Autodesk Inventor part; units mm, degrees
ref_plane "YZ Plane" through (0, 0, 0) normal (1, 0, 0) x (0, 1, 0)
ref_plane "XZ Plane" through (0, 0, 0) normal (0, 1, 0) x (-1, 0, 0)
ref_plane "XY Plane" through (0, 0, 0) normal (0, 0, 1) x (1, 0, 0)
sketch "Sketch1" plane through (0, 0, 0) normal (1, 0, 0) x (0, 1, 0)
  line L0 (6.35, -3.6662) -> (0, -7.3323)
  line L1 (0, -7.3323) -> (-6.35, -3.6662)
  line L2 (-6.35, -3.6662) -> (-6.35, 3.6662)
  line L3 (-6.35, 3.6662) -> (0, 7.3323)
  line L4 (0, 7.3323) -> (6.35, 3.6662)
  line L5 (6.35, 3.6662) -> (6.35, -3.6662)
  point P0 (0, 0)
  point P1 (0, 0)
  dimension "d0" = 6.35
extrude "Extrusion1" add sketch "Sketch1" along normal blind 3.175
sketch "Sketch3" plane through (0, 0, 0) normal (-1, 0, 0) x (0, 0, 1)
  line L0 (-3.0207, 0.0407) -> (-1.475, 2.6363)
  line L1 (-1.475, 2.6363) -> (1.5456, 2.5956)
  line L2 (1.5456, 2.5956) -> (3.0207, -0.0407)
  line L3 (3.0207, -0.0407) -> (1.475, -2.6363)
  line L4 (1.475, -2.6363) -> (-1.5456, -2.5956)
  line L5 (-1.5456, -2.5956) -> (-3.0207, 0.0407)
  line L6 (-3.6662, 6.35) -> (-7.3323, 0)
  line L7 (-7.3323, 0) -> (-3.6662, -6.35)
  line L8 (-3.6662, -6.35) -> (3.6662, -6.35)
  line L9 (3.6662, -6.35) -> (7.3323, 0)
  line L10 (7.3323, 0) -> (3.6662, 6.35)
  line L11 (3.6662, 6.35) -> (-3.6662, 6.35)
  point P0 (0, 0)
  point P1 (0, 0)
  point P2 (0, 0)
  dimension "d6" = 2.6162
extrude "Extrusion3" add sketch "Sketch3" along normal blind 12.7
extrude "Extrusion4" cut sketch "Sketch3" against normal through all contours L0 L1 L2 L3 L4 L5
properties part number "5mm-.5in hex converter"
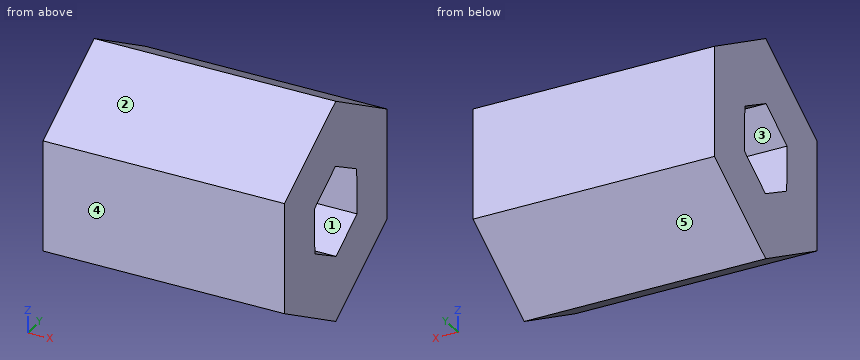
CAD build for the part. Positions are in the model's coordinates, mm. Face numbers are marked on the shaded views. A direction names the side the tool comes from. Round coordinates to 2 decimals unless told otherwise and drop trailing zeros. Write each loop counter-clockwise with the first axis right and the second up, starting at its lowest first coordinate (ties: lowest second). Pieces come first, ordered by that corner, then holes.
(1) Drop flat-ended pins along their axis: P1, Ø6, axis at x = -8, y = 1.5, coming from the -Z side; P2, Ø1.5, axis at x = -10.5, z = 4, coming from the +Y side; P3, Ø1.5, axis at x = -5.5, y = 3.5, coming from the +Z side. Give the stop position or say it passes through.
(2) Probe line 1 along Y through (x, z) = (-9, 1.5); line 2 along Z through (x, y) = (-9.75, 1.5); line 3 along Z through (x, y) = (-4.75, 2). List the from-to ranges inside material, lowest first.
(3) Slice it at A-A, the plane x = 1.5. Write the cut outline in (y, z) (3 decimals), and give its area (3 significant figures).
(4) Slice it at D-D, the plane y = -4.75. Write the cut outline in (x, z) (3 decimals), and give its area (3 significant figures).
(5) Slice it at C-C, the plane z = 0.25. Write the cut outline in (x, y) (3 decimals), and give its area (3 significant figures).
(6) Mould opens along Y. For the marked faces 3, 4 and 5 say: pulls with the +Y half, pulls with the -Y half, needs draft (parallel to the pull), parting line crosses it, or undercut.
(7) Slice it at B-B, the plane y = 1.25. Write the cut outline in (x, z) (1 decimal).
(8) 3-axis set-ups, long thin cutter, end or side, ignore diameter. For the marked faces 1 and 2: which of +Z, -Z, +X, -X, +Y, -Y reach the whole face in a straight line?
From the geometry:
1. P1: stops at z = -7.33
1. P2: stops at y = 6.35
1. P3: stops at z = 5.74
2. line 1: y = -6.35 to -2.59, 2.6 to 6.35
2. line 2: z = -6.47 to -2.15, 2.16 to 6.47
2. line 3: z = -6.18 to -1.85, 1.88 to 6.18
3. outline: (-6.35, -3.666) - (0, -7.332) - (6.35, -3.666) - (6.35, 3.666) - (0, 7.332) - (-6.35, 3.666) - close; hole (-2.636, 1.475) - (-2.596, -1.546) - (0.041, -3.021) - (2.636, -1.475) - (2.596, 1.546) - (-0.041, 3.021) - close
3. area: 116 mm2
4. outline: (-12.7, -4.59) - (3.175, -4.59) - (3.175, 4.59) - (-12.7, 4.59) - close
4. area: 146 mm2
5. outline: (-12.7, -6.35) - (3.175, -6.35) - (3.175, -2.62) - (-12.7, -2.62) - close; (-12.7, 2.613) - (3.175, 2.613) - (3.175, 6.35) - (-12.7, 6.35) - close
5. area: 119 mm2
6. face 3: undercut
6. face 4: pulls with the -Y half
6. face 5: pulls with the +Y half
7. outline: (-12.7, -6.6) - (3.2, -6.6) - (3.2, -2.3) - (-12.7, -2.3) - close; (-12.7, 2.3) - (3.2, 2.3) - (3.2, 6.6) - (-12.7, 6.6) - close
8. face 1: +X, -X
8. face 2: +Z, +X, -X, -Y
